Can you work these out from the model? Positions are in its coordinate system, mm. Face numbers are marked on the shaded views. A direction names the side the tool comes from. Round coordinates to 2 decimals unless told otherwise and drop trailing zeros. Write each loop counter-clockwise with the first axis right and the second up, starting at its lowest first coordinate (ties: lowest second). Pieces come first, ordered by that corner, then holes. Notation, with made-up numbers: (-38.5, 38.25) - (4.5, 38.25) arc R19 ccw to (4.5, 73.25) - close; hole circle Ø1 at (-14, 4.5). An arc over 180 degrees is marked (long way). One line per item, written item: value. Start each with the question number.
(1) I want a section at C-C on z = 24.5. List the corners of the cut face in (x, y) for me, plus the area to 3 significant figures.
(2) If I drill on L1, parallel to X at y = 0, z = 2.6; L2, parallel to Y at x = 0, z = 1.6; L3, parallel to Z at x = 9.5, y = -2.25, over which ranges is the centre line in solid material (lowest first)? Write a range as from..to.
(3) I want a section at A-A on y = -8. List the corners of the cut face in (x, z) for me, plus the area to 3 significant figures.
(4) On a 3-axis mill with a long thin cutter (end or side, diameter ignored), from which of +Z, -Z, +X, -X, +Y, -Y can I reach the whole of each face in a straight line? I mean the marked faces 1, 2 and 3. Say none if no direction works.
(5) I'm going to push flat-ended pins straight in: pin 1 Ø6 at (x, y) = (6, -3.5) entering from +Z; pin 2 Ø12 at (y, z) = (-5.5, 18.5) entering from +X; pin 3 Ø2 at (y, z) = (0, 20) entering from -X. Where does each tip first touch, or does it pass through?
Autodesk Inventor part; units mm, degrees
ref_plane "Plano de trabajo1" through (-11, 0, 0) normal (1, 0, 0) x (0, 1, 0)
ref_plane "XZ Plane" through (0, 0, 0) normal (0, 1, 0) x (-1, 0, 0)
ref_plane "XY Plane" through (0, 0, 0) normal (0, 0, 1) x (1, 0, 0)
sketch "Boceto1" plane through (0, 0, 0) normal (0, 0, 1) x (1, 0, 0)
  circle A0 centre (0, 0) radius 11
  dimension "DIAMETROBRIDA" = 22
extrude "Extrusión1" add sketch "Boceto1" along normal blind 4
sketch "Boceto2" plane through (0, 0, 4) normal (0, 0, 1) x (1, 0, 0)
  circle A0 centre (0, 8) radius 1.05
  circle A1 centre (-8, 0) radius 1.05
  circle A2 centre (8, 0) radius 1.05
  circle A3 centre (0, -8) radius 1.05
  circle A4 centre (0, 0) radius 11
  dimension "d7" = 2.1
  dimension "d8" = 2.1
  dimension "d9" = 2.1
  dimension "d10" = 2.1
  dimension "DistanciaBarrenos" = 8
  dimension "d31" = 8
  dimension "d32" = 8
  dimension "d33" = 8
hole "Agujero1" at (0, 8, 4) at (-8, 0, 4) at (8, 0, 4) at (0, -8, 4) direction (0, 0, -1) diameter 2.013 end through all
sketch "Boceto3" plane through (0, 0, 4) normal (0, 0, 1) x (1, 0, 0)
  circle A0 centre (0, 0) radius 6
  dimension "DIAMETROBASE" = 12
extrude "Extrusión2" add sketch "Boceto3" along normal blind 4
sketch "Boceto4" plane through (0, 0, 8) normal (0, 0, 1) x (1, 0, 0)
  arc A0 (-1.9, -3.2909) -> (-1.9, 3.2909) centre (0, 0) ccw
  line L0 (0, 0) -> (-2, 0)
  line L1 (-1.9, 3.2909) -> (-1.9, -3.2909)
  circle A1 centre (0, 0) radius 6
  dimension "DIAMETROEJE" = 7.6
  dimension "d29" = 1.9
  dimension "d38" = 2
extrude "Extrusión3" add sketch "Boceto4" along normal blind 34 contours L1 A0
ref_plane "Plano de trabajo1" through (-11, 0, 0) normal (1, 0, 0) x (0, 1, 0)
sketch "Boceto7" plane through (-11, 0, 0) normal (1, 0, 0) x (0, 1, 0)
  line L0 (0.5, 4) -> (-0.5, 4)
  line L1 (-0.5, 4) -> (-0.5, 0)
  line L2 (-0.5, 0) -> (0.5, 0)
  line L3 (0.5, 0) -> (0.5, 4)
  line L4 (0.5, 4) -> (-0.5, 0) construction
  line L5 (-0.5, 4) -> (0.5, 0) construction
  point P0 (0, 0)
  point P1 (0, 2)
  dimension "d34" = 1
  dimension "d35" = 4
extrude "Extrusión4" cut sketch "Boceto7" along normal blind 0.5
fillet "Empalme5" radius 1 2 edges at (-1.9, 0, 8) (-6, 0, 4)
equation "\"d8\" = d7"
equation "\"d9\" = d7"
equation "\"d10\" = d7"
equation "\"d29\" = 0.25 * DIAMETROEJE"
properties part number "BM-AX12" material "PETG"
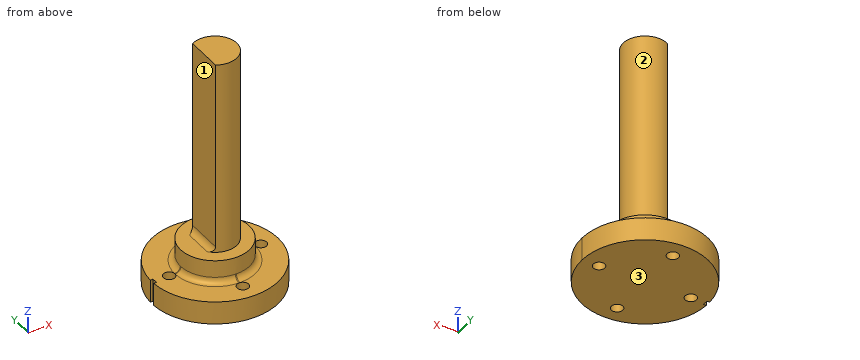
Established:
1. outline: (-1.9, -3.29) arc R3.8 ccw (long way) to (-1.9, 3.29) - close
1. area: 36.5 mm2
2. L1: -10.5..-9.01, -6.99..6.99, 9.01..11
2. L2: -11..-9.01, -6.99..6.99, 9.01..11
2. L3: 0..4
3. outline: (-7.55, 0) - (-1.01, 0) - (-1.01, 4) - (-7.55, 4) - close; (1.01, 0) - (7.55, 0) - (7.55, 4) - (1.01, 4) - close
3. area: 52.3 mm2
4. face 1: +Z, -X, +Y, -Y
4. face 2: +Z
4. face 3: -Z, +X, -X, +Y, -Y
5. pin 1: z = 8
5. pin 2: x = 3.8
5. pin 3: x = -1.9
